from build123d import *

# Parameters (mm, degrees)
SKETCH117_W             = 69.85
SKETCH117_H             = 38.1
PAD025_DEPTH            = 3.175
BODY035_PLACEMENT_ANGLE = 120


with BuildPart() as part:
    # Sketch115 → AdditiveLoft002 section 0
    with BuildSketch(Plane(origin=(-254, 0, 101.6), x_dir=(0, 1, 0), z_dir=(1, 0, 0))):
        Polygon((-38.1, 69.85), (-38.1, 0), (38.1, 0), (38.1, 69.8500000001), (34.925, 69.8500000001), (34.925, 3.175), (-34.925, 3.175), (-34.925, 69.85), align=None)
    # Sketch116 → AdditiveLoft002 section 1
    with BuildSketch(Plane(origin=(-558.8, 0, 127), x_dir=(0, 1, 0), z_dir=(1, 0, 0))):
        Polygon((-34.925, 82.55), (-34.925, 44.45), (34.925, 44.45), (34.925, 82.55), (31.75, 82.55), (31.75, 47.625), (-31.75, 47.625), (-31.75, 82.55), align=None)
    loft()

    # Sketch117 (on Face3 of AdditiveLoft002) → Pad025 (new body)
    with BuildSketch(Plane(origin=(-558.8, 0, 101.6), x_dir=(0, 1, 0), z_dir=(-1, 0, 0))):
        with Locations((0, -88.9)):
            Rectangle(SKETCH117_W, SKETCH117_H)
    extrude(amount=PAD025_DEPTH)

    # Sketch118 → Groove004 (revolve, cut)
    with BuildSketch(Plane.XZ):
        with BuildLine():
            ThreePointArc((-285.6448342114, 160.9012244898), (-330.0079117171, 85.8263739972), (-345.44, 0))
            Line((-345.44, 0), (0, 0))
            Line((0, 203.2), (0, 0))
            Line((-193.3141946016, 203.2), (0, 203.2))
            ThreePointArc((-193.3141946016, 203.2), (-244.0934556744, 192.1220184086), (-285.6448342114, 160.9012244898))
        make_face()
    revolve(axis=Axis((0, 0, 0), (1, 0, 0)), mode=Mode.SUBTRACT)


with BuildPart() as part_1:
    # Body035 placement: moved
    add(part.part.rotate(Axis((0, 0, 0), (1, 0, 0)), BODY035_PLACEMENT_ANGLE))


solid = part_1.part
CAD build for the part. Positions are in the model's coordinates, mm. A direction names the side the tool comes from. Give positions to 0.01 mm unless a question says otherwise; leave off trailing zeros. Return JSON: item names as keys, results as strings.
Item 1: Drop flat-ended pins along their axis: pin 1 (10 mm diameter, centred on x = -450.5, y = -115, fed in from +Z); pin 2 (6 mm diameter, centred on x = -507.5, z = -87.5, fed in from +Y) (3 decimals); pin 3 (6 mm diameter, centred on x = -510, y = -137.5, fed in from +Z). Give the stop position or say it passes through.
Answer below:
{"pin 1": "stops at z = -85.12", "pin 2": "stops at y = -131.975", "pin 3": "stops at z = -77"}
Item 2: Drill centre lines: probe 1 along Z at (x, y) = (-525.5, -149.5); probe 2 along Z at (x, y) = (-437, -150); probe 3 along X at (y, z) = (-169.5, -90) (3 decimals). Where is each one in solid material? Low to high.
Answer below:
{"probe 1": "z = -127.04 to -123.38, -75.05 to -68.7", "probe 2": "z = -128.4 to -124.73, -48.48 to -44.81", "probe 3": "x = -561.975 to -558.8"}
Item 3: Two-plate mould, pull along Z, no slides. Class faces 1 (the flat face through (-560.37, -181.23, -105.2)), 2 (the flat face through (-558.8, -166, -96)), 3 (the flat face through (-560.365, -148.236, -86.148)), 4 (the flat face through (-561.975, -165, -96)): +Z half, -Z half, draft (parallel to the pull), parting line (faces both ways), or undercut.
Answer below:
{"face 1": "-Z half", "face 2": "undercut", "face 3": "+Z half", "face 4": "draft"}
Item 4: Tool access for faces 5 (the flat face through (-560.37, -147.75, -125.63)), 6 (the flat face through (-560.365, -182.671, -65.137)): list every direction of +Z, -Z, +X, -X, +Y, -Y with a clear straight run to the whole face (end or side of a thin tool).
Answer below:
{"face 5": "-Z, -X, +Y", "face 6": "+Z, -X, -Y"}
